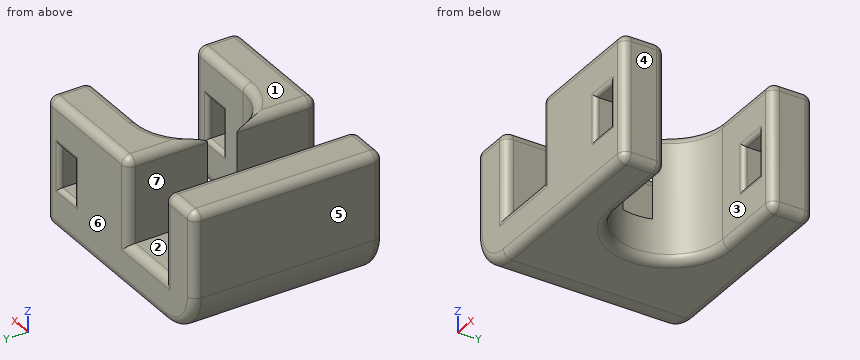
from build123d import *

# Parameters (mm, degrees)
PAD_DEPTH       = 15
SKETCH001_W     = 7
SKETCH001_H     = 22.5
POCKET_DEPTH    = 10
SKETCH002_W     = 3
SKETCH002_H     = 5
POCKET001_DEPTH = 15.001
FILLET_R        = 5
SKETCH003_W     = 3
SKETCH003_H     = 5
POCKET002_DEPTH = 22.501
FILLET001_R     = 1
FILLET002_R     = 0.5


with BuildPart() as part:
    # Sketch → Pad (new body)
    with BuildSketch(Plane.XY):
        with BuildLine():
            ThreePointArc((18.25, 17.5), (12, 11.25), (18.25, 5))
            Line((27.25, 5), (18.25, 5))
            Line((27.25, 0), (27.25, 5))
            Line((0, 0), (27.25, 0))
            Line((0, 22.5), (0, 0))
            Line((27.25, 22.5), (0, 22.5))
            Line((27.25, 17.5), (27.25, 22.5))
            Line((18.25, 17.5), (27.25, 17.5))
        make_face()
    extrude(amount=PAD_DEPTH)

    # Sketch001 (on Face10 of Pad) → Pocket (cut)
    with BuildSketch(Plane.XY.offset(15)):
        with Locations((8.75, 11.25)):
            Rectangle(SKETCH001_W, SKETCH001_H)
    extrude(amount=-POCKET_DEPTH, mode=Mode.SUBTRACT)

    # Sketch002 (on Face8 of Pocket) → Pocket001 (cut, through all)
    with BuildSketch(Plane.XY.offset(15)):
        with Locations((28.5, 7.5)):
            Rectangle(SKETCH002_W, SKETCH002_H)
    extrude(amount=-POCKET001_DEPTH, mode=Mode.SUBTRACT)

    # Fillet
    fillet_edges = [part.edges().sort_by_distance(p)[0] for p in [
        (0, 11.25, 0),
    ]]
    fillet(fillet_edges, radius=FILLET_R)

    # Sketch003 (on Face2 of Fillet) → Pocket002 (cut, through all)
    with BuildSketch(Plane.XZ):
        with Locations((23.5, 7.5)):
            Rectangle(SKETCH003_W, SKETCH003_H)
    extrude(amount=-POCKET002_DEPTH, mode=Mode.SUBTRACT)

    # Fillet001
    fillet001_edges = [part.edges().sort_by_distance(p)[0] for p in [
        (2.625, 0, 15),
        (0, 11.25, 15),
        (5.25, 11.25, 15),
        (2.625, 22.5, 15),
        (19.75, 0, 15),
        (27.25, 2.5, 15),
        (27.25, 0, 7.5),
        (16.125, 0, 0),
        (12.25, 4.75, 15),
        (27.25, 2.5, 0),
        (5.25, 0, 10),
        (12.25, 0, 10),
        (8.75, 0, 5),
        (27.25, 5, 7.5),
        (27.25, 17.5, 7.5),
        (27.25, 20, 0),
        (27.25, 22.5, 7.5),
        (27.25, 20, 15),
        (19.75, 22.5, 15),
        (12.25, 17.75, 15),
        (16.125, 22.5, 0),
        (12.25, 22.5, 10),
        (5.25, 22.5, 10),
        (0, 22.5, 10),
        (8.75, 22.5, 5),
        (1.464466, 22.5, 1.464466),
        (22.625, 5, 0),
        (12, 11.25, 0),
        (22.75, 17.5, 0),
        (22.625, 5, 15),
        (14.5, 6.25, 15),
        (14.5, 16.25, 15),
        (22.75, 17.5, 15),
    ]]
    fillet(fillet001_edges, radius=FILLET001_R)

    # Fillet002
    fillet002_edges = [part.edges().sort_by_distance(p)[0] for p in [
        (22, 0, 7.5),
        (23.5, 0, 10),
        (25, 0, 7.5),
        (23.5, 0, 5),
        (23.5, 17.5, 10),
        (22, 17.5, 7.5),
        (23.5, 17.5, 5),
        (25, 17.5, 7.5),
        (23.5, 5, 10),
        (22, 5, 7.5),
        (23.5, 5, 5),
        (25, 5, 7.5),
        (22, 22.5, 7.5),
        (23.5, 22.5, 10),
        (25, 22.5, 7.5),
        (23.5, 22.5, 5),
    ]]
    fillet(fillet002_edges, radius=FILLET002_R)


solid = part.part
Geometry: final body of the model. Coordinates: model frame, mm. Face numbers are marked on the shaded views. A direction names the side the tool comes from. Coordinates: 2 decimals unless noted, no trailing zeros. Order: outer loops, then holes, each group sorted by start corner. A loop starts at its lowest first (then second) coordinate and runs counter-clockwise, first axis right, second up.
1) Section D-D (z = 9.25). Give the number of separate pieces and of enclosed holes in the cut face, then the cut area to 3 significant figures.
Result sheet:
separate pieces: 5
enclosed holes: 0
area: 250 mm2
2) Draft query along X for the marked faces 4, 5, 6 and 7. Return one class per face: released by +X, released by -X, zero draft, split by the parting line, or undercut.
Result sheet:
face 4: released by +X
face 5: released by -X
face 6: zero draft
face 7: undercut
3) Section B-B (z = 13.5). Return loops of the section in (x, y).
Result sheet:
outline: (0, 1) arc R1 ccw to (1, 0) - (4.25, 0) arc R1 ccw to (5.25, 1) - (5.25, 21.5) arc R1 ccw to (4.25, 22.5) - (1, 22.5) arc R1 ccw to (0, 21.5) - close; (12.25, 1) arc R1 ccw to (13.25, 0) - (26.25, 0) arc R1 ccw to (27.25, 1) - (27.25, 4) arc R1 ccw to (26.25, 5) - (18.25, 5) arc R6.25 cw to (12.25, 9.5) - close; (12.25, 13) arc R6.25 cw to (18.25, 17.5) - (26.25, 17.5) arc R1 ccw to (27.25, 18.5) - (27.25, 21.5) arc R1 ccw to (26.25, 22.5) - (13.25, 22.5) arc R1 ccw to (12.25, 21.5) - close
4) Ray query, probe 1 along X at (y, z) = (18.5, 7.75); probe 2 along Y at (x, z) = (22, 13.75); probe 3 along Z at (x, y) = (22.25, 4). Return the intervals inside material, ascending.
Result sheet:
probe 1: x = 0 to 5.25, 12.25 to 22, 25 to 27.25
probe 2: y = 0 to 5, 17.5 to 22.5
probe 3: z = 0 to 5, 10 to 15
5) Set-up query: the marked faces 1, 2 and 3. Return all of +Z, -Z, +X, -X, +Y, -Y with unobstructed straight access to the full face (end or side cutting, diameter ignored); none if empty.
Result sheet:
face 1: +Z, +X, -X, +Y, -Y
face 2: +Z, +Y, -Y
face 3: +Z, -Z, +X
6) First-contact query: P1, Ø2.5, axis at y = 9, z = 10, coming from the +X side; P2, Ø4, axis at y = 6.5, z = 13, coming from the +X side. Flat tips, straight axial feed; report the tip coordinate or a pass-through.
Result sheet:
P1: stops at x = 13.07
P2: stops at x = 27.12
7) Section C-C (x = 8.75). Return loops of the section in (y, z), then the cut area to 3 significant figures.
Result sheet:
outline: (0, 1) arc R1 ccw to (1, 0) - (21.5, 0) arc R1 ccw to (22.5, 1) - (22.5, 4) arc R1 ccw to (21.5, 5) - (1, 5) arc R1 ccw to (0, 4) - close
area: 112 mm2
8) Section A-A (y = 3.5). Return loops of the section in (x, z), then the cut area to 3 significant figures.
Result sheet:
outline: (0, 5) arc R5 ccw to (5, 0) - (26.25, 0) arc R1 ccw to (27.25, 1) - (27.25, 14) arc R1 ccw to (26.25, 15) - (13.25, 15) arc R1 ccw to (12.25, 14) - (12.25, 5) - (5.25, 5) - (5.25, 14) arc R1 ccw to (4.25, 15) - (1, 15) arc R1 ccw to (0, 14) - close; hole (22, 5) - (25, 5) - (25, 10) - (22, 10) - close
area: 317 mm2
